Part print with two shaded views. Sizes in mm from the minimum x, y, z corner. A direction names the side the tool comes from. Round coordinates to 2 decimals unless told otherwise and drop trailing zeros. Order: outer loops, then holes, each group sorted by start corner. A loop starts at its lowest first (then second) coordinate and runs counter-clockwise, first axis right, second up. Notation, with made-up numbers: (-17, 33.5) -> (-1, 33.5) arc R16 cw to (-1, 39.5) -> close; hole circle Ø9 at (86, -6.5). An arc over 180 degrees is marked (long way). Put each result on its own line as item: value. Start each with the question number.
Q1. 3-axis set-ups, long thin cutter, end or side, ignore diameter. For the marked faces 1 and 2: which of +Z, -Z, +X, -X, +Y, -Y reach the whole face in a straight line?
Q2. Probe L1, parallel to Y at x = 25, z = 2.15; L2, parallel to Y at x = 25, z = 21.5; L3, parallel to Z at x = 45, y = 34.5. List the from-to ranges inside material, lowest first.
Q3. Cut at A-A, the plane y = 25. List the corners of the cut face in (x, z).
Q4. Flat gauge pins, fed straight in: P1, Ø3.5, axis at x = 37.12, y = 32, coming from the +Z side; P2, Ø4, axis at x = 7, z = 3.5, coming from the -Y side; P3, Ø12, axis at y = 32.5, z = 13, coming from the +X side; P4, Ø2.5, axis at x = 12.88, y = 18, coming from the +Z side. Where does each tip first touch, or does it go through?
Q5. Cut at C-C, the plane y = 39. List the corners of the cut face in (x, z), and give its area (3 significant figures).
Q6. Cut at D-D, the plane z = 10.75. List the corners of the cut face in (x, y).
Q7. Cut at B-B, the plane x = 25. List the corners of the cut face in (y, z), and give its area (3 significant figures).
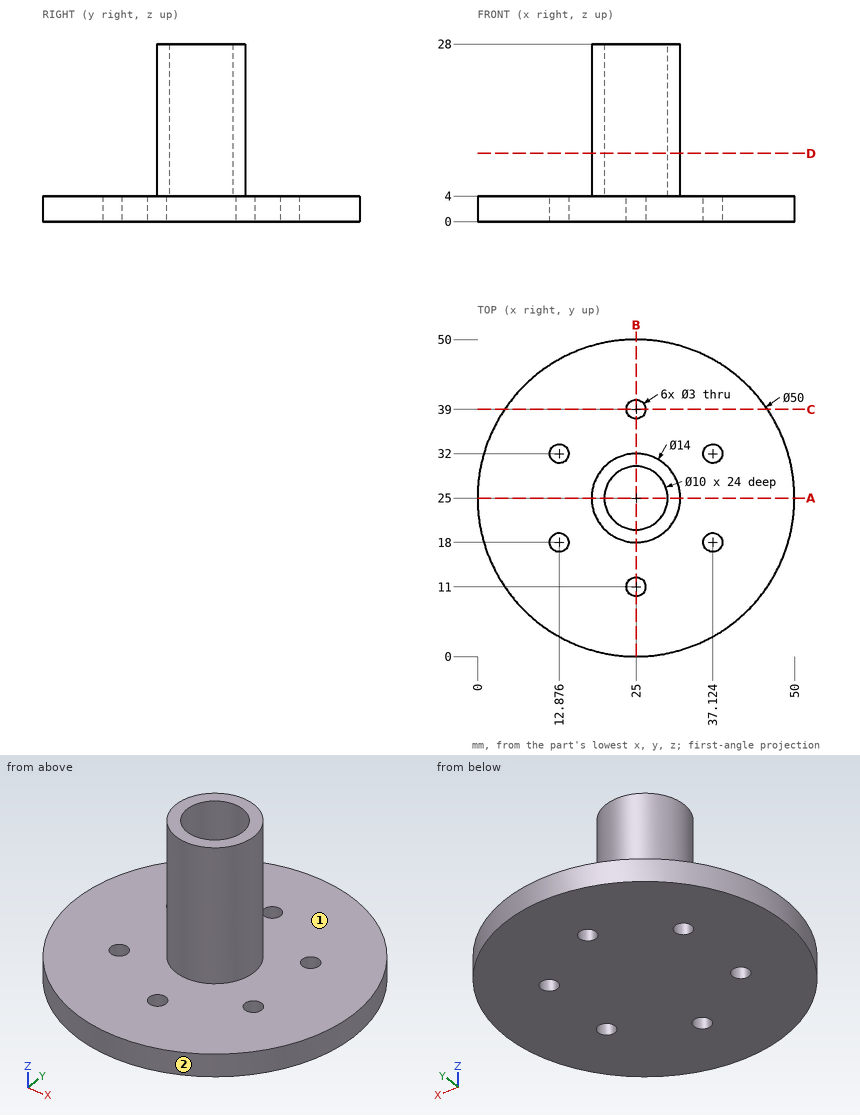
Ans:
1. face 1: +Z
1. face 2: +Z, -Z
2. L1: y = 0 to 9.5, 12.5 to 37.5, 40.5 to 50
2. L2: y = 18 to 20, 30 to 32
2. L3: z = 0 to 4
3. outline: (0, 0) -> (50, 0) -> (50, 4) -> (32, 4) -> (32, 28) -> (30, 28) -> (30, 4) -> (20, 4) -> (20, 28) -> (18, 28) -> (18, 4) -> (0, 4) -> close
4. P1: stops at z = 4
4. P2: stops at y = 5.79
4. P3: stops at x = 31.84
4. P4: passes through
5. outline: (4.29, 0) -> (23.5, 0) -> (23.5, 4) -> (4.29, 4) -> close; (26.5, 0) -> (45.71, 0) -> (45.71, 4) -> (26.5, 4) -> close
5. area: 154 mm^2
6. outline: circle Ø14 at (25, 25); hole circle Ø10 at (25, 25)
7. outline: (0, 0) -> (9.5, 0) -> (9.5, 4) -> (0, 4) -> close; (12.5, 0) -> (37.5, 0) -> (37.5, 4) -> (32, 4) -> (32, 28) -> (30, 28) -> (30, 4) -> (20, 4) -> (20, 28) -> (18, 28) -> (18, 4) -> (12.5, 4) -> close; (40.5, 0) -> (50, 0) -> (50, 4) -> (40.5, 4) -> close
7. area: 272 mm^2
